Input: part model. Units: mm. Frame: model coordinates. A direction names the side the tool comes from. Coordinates: 2 decimals unless noted, no trailing zeros. Write each loop counter-clockwise with the first axis right and the second up, starting at its lowest first coordinate (ties: lowest second). Pieces come first, ordered by that corner, then holes. Notation, with made-up numbers: (-11.75, 12.5) - (23.25, 12.5) arc R21 ccw to (23.25, 22.5) - close; hole circle Ø5 at (84, 7.25). An arc over 180 degrees is marked (long way). Use a Markdown table: item, result. Add a question column.
Q1. Section query B-B (y = 45). Return the cut outline in (x, z) (3 decimals).
Q2. Pin query (flat end, axial travel): P1, Ø4, axis at x = -41.5, z = 57, coming from the +Y side; P2, Ø19.5, axis at y = 59.5, z = 32, coming from the -X side. Return the tip coordinate at first contact, or that it passes through.
Q3. Set-up query: faces 1 (the face through (-52, -7, 39)), 2 (the face through (-45, 0, 32)). Return all of +Z, -Z, +X, -X, +Y, -Y with unobstructed straight access to the full face (end or side cutting, diameter ignored); none if empty.
Q4. Section query D-D (z = 60). Return the cut outline in (x, y), then the cut area to 3 significant figures.
Q5. Mould query, pull axis Z, two halves, no side actions, for faces 3 (the face through (-52.72, -3.55, 36.37)), 4 (the face through (-110, -3, 32)), 5 (the face through (-26, -1, 0)), 6 (the face through (3.549, 32.137, 33.066)). Classes: released by +Z, released by -Z, zero draft, split by the parting line, or undercut.
Q6. Section query A-A (x = -65). Return the cut outline in (y, z) (3 decimals), then the cut area to 3 significant figures.
Q7. Section query C-C (z = 32.5). Return the cut outline in (x, y) (3 decimals), then the cut area to 3 significant figures.
Q8. Material intervals for probe 1 along Z at (x, y) = (-65, -5.5) (3 decimals); probe 2 along Y at (x, z) = (5, 32); probe 3 along X at (y, z) = (5, 22), sorted ascending. Write a range as from..to.
from build123d import *

# Parameters (mm, degrees)
F1_DEPTH = 65
F2_R     = 5
F3_R     = 12.875
F4_DEPTH = 7
F5_R     = 12.875
F6_DEPTH = 7


with BuildPart() as f1:
    # F0 (on Top) → F1 (new body)
    with BuildSketch(Plane.XY):
        Polygon((0, 0), (-110, 0), (-110, -7), (7, -7), (7, 90), (0, 90), align=None)
    extrude(amount=F1_DEPTH)

    # F2
    f2_edges = [f1.edges().sort_by_distance(p)[0] for p in [
        (0, 0, 32.5),
    ]]
    fillet(f2_edges, radius=F2_R)

    # F3 (on face) → F4 (cut)
    with BuildSketch(Plane.YZ.offset(7)):
        with Locations((45, 32.5)):
            Circle(F3_R)
    extrude(amount=-F4_DEPTH, mode=Mode.SUBTRACT)

    # F5 (on face) → F6 (cut)
    with BuildSketch(Plane.XZ.offset(7)):
        with Locations((-65, 32.5)):
            Circle(F5_R)
    extrude(amount=-F6_DEPTH, mode=Mode.SUBTRACT)


solid = f1.part
Values follow:
| question | item | result |
|---|---|---|
| 1 | outline | (0, 0) - (7, 0) - (7, 19.625) - (0, 19.625) - close; (0, 45.375) - (7, 45.375) - (7, 65) - (0, 65) - close |
| 2 | P1 | y = 0 |
| 2 | P2 | x = 0 |
| 3 | face 1 | +Z, -Z, +X, -X, -Y |
| 3 | face 2 | +Z, -Z, -X, +Y |
| 4 | outline | (-110, -7) - (7, -7) - (7, 90) - (0, 90) - (0, 5) arc R5 cw to (-5, 0) - (-110, 0) - close |
| 4 | area | 1,450 mm2 |
| 5 | face 3 | undercut |
| 5 | face 4 | zero draft |
| 5 | face 5 | released by -Z |
| 5 | face 6 | undercut |
| 6 | outline | (-7, 0) - (0, 0) - (0, 19.625) - (-7, 19.625) - close; (-7, 45.375) - (0, 45.375) - (0, 65) - (-7, 65) - close |
| 6 | area | 275 mm2 |
| 7 | outline | (-110, -7) - (-77.875, -7) - (-77.875, 0) - (-110, 0) - close; (-52.125, -7) - (7, -7) - (7, 32.125) - (0, 32.125) - (0, 5) arc R5 cw to (-5, 0) - (-52.125, 0) - close; (0, 57.875) - (7, 57.875) - (7, 90) - (0, 90) - close |
| 7 | area | 1,090 mm2 |
| 8 | probe 1 | 0..19.625, 45.375..65 |
| 8 | probe 2 | -7..32.13, 57.87..90 |
| 8 | probe 3 | 0..7 |
